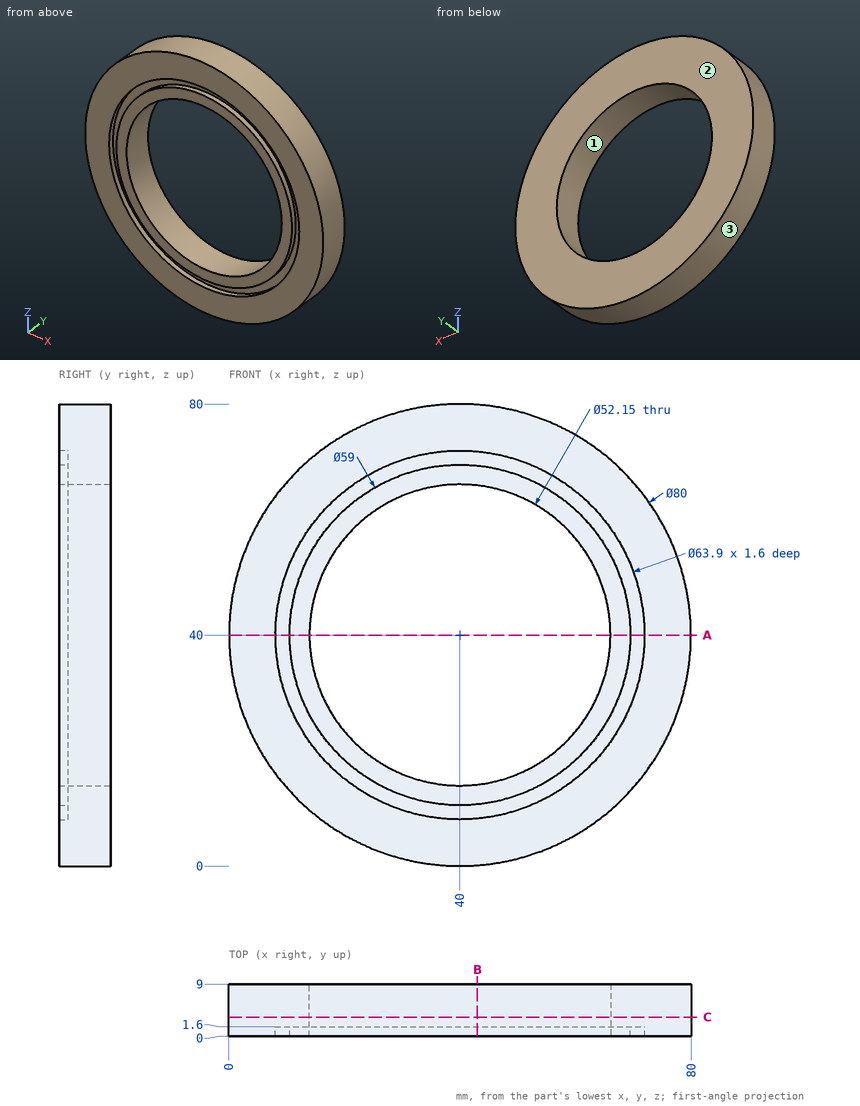
Job drawing, mm, ordinate dimensions from the low corner. One solid piece. Coordinates: 2 decimals unless noted, no trailing zeros. Order: outer loops, then holes, each group sorted by start corner. A loop starts at its lowest first (then second) coordinate and runs counter-clockwise, first axis right, second up. Notation, with made-up numbers: (68.5, -34.75) - (121.5, -34.75) arc R17 cw to (121.5, -7.75) - close; hole circle Ø2 at (16, -14.5). An arc over 180 degrees is marked (long way). Write each question's results on one line, items separated by ' | '. Start each with the question number.
Item 1: Band-saw the part on C-C on y = 3.25. Write the cut outline in (x, z) (3 decimals).
Item 2: Flat gauge pins, fed straight in: pin 1 (3 mm diameter, centred on x = 47, y = 4, fed in from -Z); pin 2 (2 mm diameter, centred on x = 54.5, y = 2.5, fed in from +Z); pin 3 (1.5 mm diameter, centred on y = 8, z = 31, fed in from -X). Where does each tip first touch, or does it go through?
Item 3: Band-saw the part on B-B on x = 43. Write the cut outline in (y, z), and give its area (3 significant figures).
Item 4: Mould opens along Z. For the marked faces 1, 2 and 3 say: released by +Z, released by -Z, zero draft, split by the parting line, or undercut.
Item 5: Wall check: probe 1 along Z at (x, y) = (40, 0.4) (3 decimals); probe 2 along Z at (x, y) = (40, 5.5) (3 decimals); probe 3 along X at (y, z) = (5, 37). Give the ranges that are in metal, low to high. Write a range as [from, to].
Item 6: Band-saw the part on A-A on z = 40. Write the cut outline in (x, y) (3 decimals).
Numbers:
1) outline: circle Ø80 at (40, 40); hole circle Ø52.15 at (40, 40)
2) pin 1: z = 0.38 | pin 2: z = 77.65 | pin 3: x = 0.86
3) outline: (0, 0.11) - (9, 0.11) - (9, 14.1) - (0, 14.1) - (0, 10.65) - (1.6, 10.65) - (1.6, 8.19) - (0, 8.19) - close; (0, 65.9) - (9, 65.9) - (9, 79.89) - (0, 79.89) - (0, 71.81) - (1.6, 71.81) - (1.6, 69.35) - (0, 69.35) - close | area: 244 mm^2
4) face 1: undercut | face 2: zero draft | face 3: split by the parting line
5) probe 1: [0, 8.05], [10.5, 13.925], [66.075, 69.5], [71.95, 80] | probe 2: [0, 13.925], [66.075, 80] | probe 3: [0.11, 14.1], [65.9, 79.89]
6) outline: (0, 0) - (8.05, 0) - (8.05, 1.6) - (10.5, 1.6) - (10.5, 0) - (13.925, 0) - (13.925, 9) - (0, 9) - close; (66.075, 0) - (69.5, 0) - (69.5, 1.6) - (71.95, 1.6) - (71.95, 0) - (80, 0) - (80, 9) - (66.075, 9) - close
